CAD build for the part. Positions are in the model's coordinates, mm. Face numbers are marked on the shaded views. A direction names the side the tool comes from. Coordinates: 2 decimals unless noted, no trailing zeros. Loops run counter-clockwise (first coordinate to the right, second up) from the corner with the lowest first, then second, coordinate; pieces in that order, holes last. Notation, with made-up numbers: (-5, 57.25) -> (28, 57.25) arc R29 cw to (28, 78.25) -> close; hole circle Ø4 at (34, 37). An arc over 180 degrees is marked (long way). Return JSON: item names as keys, results as strings. Group by question number.
(1) Mould opens along X. For the marked faces 4 and 5 say: pulls with the +X half, pulls with the -X half, needs draft (parallel to the pull), parting line crosses it, or undercut.
(2) Saw through at A-A on z = -15. Write the cut outline in (x, y).
(3) Flat gauge pins, fed straight in: pin 1 Ø0.9 at (x, z) = (-4.25, 0) entering from -Y; pin 2 Ø0.6 at (x, y) = (4, 10) entering from +Z; pin 3 Ø3 at (y, z) = (31, -30) entering from -X; pin 4 Ø4 at (x, z) = (-29, 39) entering from +Y. Where does each tip first touch, or does it go through?
(4) Probe L1, parallel to X at y = 7.5, z = 0; L2, parallel to Y at x = 7, z = 10.5; L3, parallel to X at y = 11.5, z = -25. List the from-to ranges inside material, lowest first.
(5) Saw through at D-D on x = -37.5. Write the cut outline in (y, z), then the cut area to 3 significant figures.
(6) Saw through at B-B on y = 16. Write the cut outline in (x, z).
(7) Saw through at C-C on x = 43.5. Write the cut outline in (y, z), then the cut area to 3 significant figures.
(8) Tool access for the marked faces 1, 2 and 3: list every direction of +Z, -Z, +X, -X, +Y, -Y with a clear straight run to the whole face (end or side of a thin tool).
```python
from build123d import *

# Parameters (mm, degrees)
SKETCH1_R               = 50.9
BOSS_EXTRUDE1_DEPTH     = 10
BOSS_EXTRUDE2_DEPTH     = 40
SKETCH3_W               = 40
SKETCH3_H               = 20
CUT_EXTRUDE1_DEPTH      = 0.5
CUT_EXTRUDE2_DEPTH      = 113.361247768
CUT_EXTRUDE2_DEPTH_BACK = 113.361247768
SKETCH4_R               = 2.5
SKETCH5_R               = 0.75
CUT_EXTRUDE3_DEPTH      = 88.644851647


with BuildPart() as part:
    # Sketch1 → Boss-Extrude1 (new body)
    with BuildSketch(Plane(origin=(0, 0, 0), x_dir=(1, 0, 0), z_dir=(0, 1, 0))):
        with Locations(Location((0, 0, 0), (0, 0, 270))):
            Circle(SKETCH1_R)
    extrude(amount=BOSS_EXTRUDE1_DEPTH)

    # Sketch2 → Boss-Extrude2 (add)
    with BuildSketch(Plane(origin=(0, 10, 0), x_dir=(1, 0, 0), z_dir=(0, 1, 0))):
        with BuildLine():
            Line((-35.9, 36.083237105), (-35.9, -36.083237105))
            ThreePointArc((-35.9, -36.083237105), (-50.9, 0), (-35.9, 36.083237105))
        make_face()
        with BuildLine():
            Line((35.9, 36.083237105), (35.9, -36.083237105))
            ThreePointArc((35.9, -36.083237105), (50.9, 0), (35.9, 36.083237105))
        make_face()
    extrude(amount=BOSS_EXTRUDE2_DEPTH)

    # Sketch3 → Cut-Extrude1 (cut)
    with BuildSketch(Plane(origin=(0, 10, 0), x_dir=(1, 0, 0), z_dir=(0, 1, 0))):
        Rectangle(SKETCH3_W, SKETCH3_H)
    extrude(amount=-CUT_EXTRUDE1_DEPTH, mode=Mode.SUBTRACT)

    # Sketch4 → Cut-Extrude2 (cut, two sides: drawn at the far end of the back side and taken through both)
    with BuildSketch(Plane.ZY.offset(-35.9).offset(-CUT_EXTRUDE2_DEPTH_BACK)):
        with Locations(Location((0, 40, 0), (0, 0, 270))):
            Circle(SKETCH4_R)
    extrude(amount=CUT_EXTRUDE2_DEPTH + CUT_EXTRUDE2_DEPTH_BACK, mode=Mode.SUBTRACT)

    # Sketch5 → Cut-Extrude3 (cut, through all)
    with BuildSketch(Plane.XZ):
        with Locations(Location((-4.25, 0, 0), (0, 0, 270))):
            Circle(SKETCH5_R)
        with Locations(Location((0, 4.25, 0), (0, 0, 270))):
            Circle(SKETCH5_R)
        with Locations(Location((4.25, 0, 0), (0, 0, 270))):
            Circle(SKETCH5_R)
        with Locations(Location((0, -4.25, 0), (0, 0, 270))):
            Circle(SKETCH5_R)
    extrude(amount=-CUT_EXTRUDE3_DEPTH, mode=Mode.SUBTRACT)


solid = part.part
```
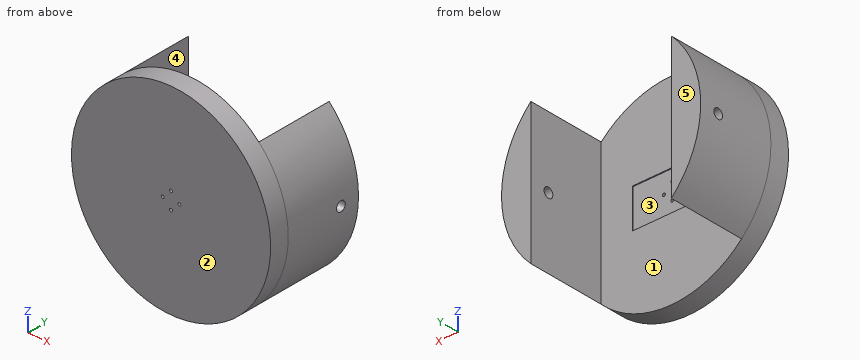
Geometry results:
{
 "1": {"face 4": "undercut", "face 5": "needs draft"},
 "2": {"outline": "(-48.64, 0) -> (48.64, 0) -> (48.64, 50) -> (35.9, 50) -> (35.9, 10) -> (-35.9, 10) -> (-35.9, 50) -> (-48.64, 50) -> close"},
 "3": {"pin 1": "through", "pin 2": "z = 50.77", "pin 3": "x = -42.17", "pin 4": "y = 10"},
 "4": {"L1": "-50.9 to -5, -3.5 to 3.5, 5 to 50.9", "L2": "0 to 10", "L3": "-44.34 to -35.9, 35.9 to 44.34"},
 "5": {"outline": "(0, -34.42) -> (50, -34.42) -> (50, 34.42) -> (0, 34.42) -> close; hole circle Ø5 at (40, 0)", "area": "3,420 mm²"},
 "6": {"outline": "(-35.9, -36.08) -> (-35.9, 36.08) arc R50.9 ccw to start; (35.9, -36.08) arc R50.9 ccw to (35.9, 36.08) -> close"},
 "7": {"outline": "(0, -26.43) -> (50, -26.43) -> (50, 26.43) -> (0, 26.43) -> close; hole circle Ø5 at (40, 0)", "area": "2,620 mm²"},
 "8": {"face 1": "+Z, -Z, +Y", "face 2": "+Z, -Z, +X, -X, -Y", "face 3": "+Y"}
}
